CAD build for the part. Positions are in the model's coordinates, mm. A direction names the side the tool comes from. Give positions to 0.01 mm unless a question says otherwise; leave off trailing zeros. Write each loop counter-clockwise with the first axis right and the second up, starting at its lowest first coordinate (ties: lowest second). Pieces come first, ordered by that corner, then holes. Notation, with made-up numbers: (47, 52.5) - (65, 52.5) arc R18 ccw to (65, 79.5) - close; hole circle Ø10 at (21.5, -20.75). An arc over 180 degrees is marked (long way). Put each result on its own line as item: value. Start each with the question number.
1. Wall check: line 1 (Z direction, x = 2, y = -24.5); line 2 (Y direction, x = 1.15, z = -25.25); line 3 (Y direction, x = 2.3, z = -25.25). Give the ranges that are in metal, low to high.
2. Cut at A-A on x = 10.5. List the corners of the cut face in (y, z).
3. Drop flat-ended pins along their axis: pin 1 (2 mm diameter, centred on x = 9, z = 50.5, fed in from +Y); pin 2 (13.5 mm diameter, centred on y = 25.25, z = -25.25, fed in from +X); pin 3 (1.5 mm diameter, centred on x = 7.5, y = -17.5, fed in from -Z). Give the stop position or say it passes through.
4. Mould opens along Y. For faces 3 (the cylindrical face through (7.437, -1.099, 69.988)), 4 (the flat face through (8, -47, 0)), 5 (the cylindrical face through (0.9, -49.14, -0.28)) say: +Y half, -Y half, draft (parallel to the pull), parting line (faces both ways), or undercut.
5. Cut at D-D on z = 25.25. Give the number of separate pieces and of enclosed holes in the cut face, and give its area (3 significant figures).
6. Tool access for faces 1 (the cylindrical face through (7.56, 1.03, 66.99)), 2 (the cylindrical face through (7.437, 1.099, -69.988)): list every direction of +Z, -Z, +X, -X, +Y, -Y with a clear straight run to the whole face (end or side of a thin tool).
7. Cut at C-C on y = 0. List the corners of the cut face in (x, z), and give its area (3 significant figures).
8. Cut at B-B on z = -14. List the corners of the cut face in (x, y).
Autodesk Inventor part; units mm, degrees
ref_plane "YZ Plane" through (0, 0, 0) normal (1, 0, 0) x (0, 1, 0)
ref_plane "XZ Plane" through (0, 0, 0) normal (0, 1, 0) x (-1, 0, 0)
ref_plane "XY Plane" through (0, 0, 0) normal (0, 0, 1) x (1, 0, 0)
sketch "Náčrt1" plane through (0, 0, 0) normal (1, 0, 0) x (0, 1, 0)
  line L0 (50, 70) -> (-50, 70)
  line L1 (-50, 70) -> (-50, -70)
  line L2 (-50, -70) -> (50, -70)
  line L3 (50, -20) -> (50, 70)
  arc A0 (50, 20) -> (-50, 20) centre (0, 20) ccw
  arc A1 (-50, -20) -> (50, -20) centre (0, -20) ccw
  point P0 (0, 0)
  dimension "d0" = 100
  dimension "d1" = 140
  dimension "d2" = 50
  dimension "d3" = 70
  dimension "d4" = 100
  dimension "d8" = 100
extrude "Vysunutí2" add sketch "Náčrt1" along normal blind 12 contours A0 L3 A1 L1
sketch "Náčrt2" plane through (12, 0, 0) normal (1, 0, 0) x (0, 0, -1)
  arc A0 (-20, 50) -> (-20, -50) centre (-20, 0) ccw
  line L0 (-20, -50) -> (20, -50)
  arc A1 (20, -50) -> (20, 50) centre (20, 0) ccw
  line L1 (20, 50) -> (-20, 50)
  arc A2 (-20, 47) -> (-20, -47) centre (-20, 0) ccw
  line L2 (-20, -47) -> (20, -47)
  arc A3 (20, -47) -> (20, 47) centre (20, 0) ccw
  line L3 (20, 47) -> (-20, 47)
  point P0 (0, 0)
  dimension "d11" = 3
extrude "Vysunutí3" cut sketch "Náčrt2" against normal blind 9 contours L3 A3 L2 A2
sketch "Náčrt4" plane through (0, 0, 0) normal (-1, 0, 0) x (0, 0, 1)
  circle A0 centre (25.25, -25.25) radius 4.25
  arc A1 (20, -50) -> (20, 50) centre (20, 0) ccw
  line L0 (-20, 50) -> (20, 50)
  arc A2 (-20, 50) -> (-20, -50) centre (-20, 0) ccw
  line L1 (20, -50) -> (-20, -50)
  arc A3 (20, -50) -> (20, 50) centre (20, 0) ccw
  circle A4 centre (25.25, 25.25) radius 4.25
  circle A5 centre (-25.25, 25.25) radius 4.25
  circle A6 centre (-25.25, -25.25) radius 4.25
  point P0 (0, 0)
  point P1 (70, 0)
  dimension "d25" = 8.5
  dimension "d26" = 24.75
  dimension "d27" = 44.75
  dimension "d32" = 360
extrude "Vysunutí5" cut sketch "Náčrt4" against normal through all contours A0 | A4 | A5 | A6
fillet "Zaoblení2" radius 3 4 edges at (0, -50, 0) (0, 0, -70) (0, 50, 0) (0, 0, 70)
properties part number "Anténní držák"
Report:
1. line 1: z = -63.39 to -29.43, -21.07 to 21.07, 29.43 to 63.39
1. line 2: y = -49.08 to -29.5, -21 to 21, 29.5 to 49.08
1. line 3: y = -49.64 to -29.5, -21 to 21, 29.5 to 49.64
2. outline: (-50, -20) arc R50 ccw to (50, -20) - (50, 20) arc R50 ccw to (-50, 20) - close; hole (-47, -20) arc R47 ccw to (47, -20) - (47, 20) arc R47 ccw to (-47, 20) - close
3. pin 1: stops at y = 40.37
3. pin 2: stops at x = 3
3. pin 3: stops at z = -67.11
4. face 3: parting line
4. face 4: undercut
4. face 5: -Y half
5. separate pieces: 3
5. enclosed holes: 0
5. area: 298 mm²
6. face 1: +X
6. face 2: -Z, +X, -X
7. outline: (0, -67) arc R3 ccw to (3, -70) - (12, -70) - (12, -67) - (3, -67) - (3, 67) - (12, 67) - (12, 70) - (3, 70) arc R3 ccw to (0, 67) - close
7. area: 470 mm²
8. outline: (0, -47) arc R3 ccw to (3, -50) - (12, -50) - (12, -47) - (3, -47) - (3, 47) - (12, 47) - (12, 50) - (3, 50) arc R3 ccw to (0, 47) - close
